Geometry: final body of the model. Coordinates: model frame, mm. Face numbers are marked on the shaded views. A direction names the side the tool comes from. Coordinates: 2 decimals unless noted, no trailing zeros. Write each loop counter-clockwise with the first axis right and the second up, starting at its lowest first coordinate (ties: lowest second). Pieces come first, ordered by that corner, then holes. Notation, with made-up numbers: (-22.75, 60) - (30.25, 60) arc R19 cw to (30.25, 69) - close; hole circle Ø2 at (82, -25). An arc over 180 degrees is marked (long way). Answer as a JSON object with one key per item and string values. Group by question number.
Item 1: First-contact query: pin 1 Ø1.5 at (y, z) = (6.5, 1) entering from +X; pin 2 Ø10 at (x, y) = (0, 0) entering from -Z; pin 3 Ø9.5 at (x, y) = (0, 18.97) entering from -Z; pin 4 Ø3.5 at (y, z) = (26, 3) entering from +X. Flat tips, straight axial feed; report the tip coordinate or a pass-through.
Item 2: Set-up query: the marked faces 5, 6 and 7. Return all of +Z, -Z, +X, -X, +Y, -Y with unobstructed straight access to the full face (end or side cutting, diameter ignored); none if empty.
Item 3: Mould query, pull axis X, two halves, no side actions, for the marked faces 1, 2, 3 and 4. Classes: pulls with the +X half, pulls with the -X half, needs draft (parallel to the pull), parting line crosses it, or undercut.
Item 4: Section A-A on y = 34. Return loops of the section in (x, z).
Item 5: Section B-B on z = 1. State how many separate pieces and enclosed holes the cut face has, and give its area (3 significant figures).
Item 6: Line query: line 1 along Y through (x, z) = (0, 5); line 2 along X through (y, z) = (-4, 6); line 3 along X through (y, z) = (-1, 0.5). Output: solid intervals per line, ascending. Write a range as from..to.
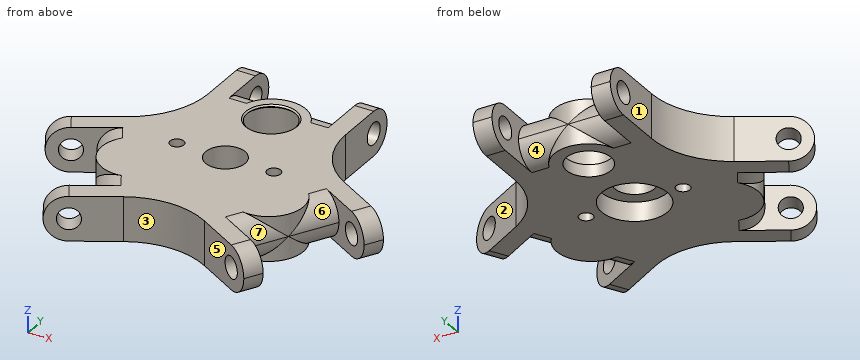
```python
from build123d import *

# Parameters (mm, degrees)
SKETCH1_R           = 8.15
BOSS_EXTRUDE1_DEPTH = 11
FILLET1_R           = 5.5
SKETCH5_R           = 8.534526782
BOSS_EXTRUDE2_DEPTH = 11
SKETCH6_R           = 8.534526782
BOSS_EXTRUDE3_DEPTH = 11
SKETCH7_R           = 8.534526782
BOSS_EXTRUDE4_DEPTH = 11
SKETCH8_R           = 1.7
CUT_EXTRUDE4_DEPTH  = 58.906789501
BOSS_EXTRUDE5_START = -6.25
SKETCH12_R          = 8.15
BOSS_EXTRUDE5_DEPTH = 6.25
SKETCH14_R          = 4.8895
CUT_EXTRUDE7_DEPTH  = 58.906789501
SKETCH15_R          = 6.7
CUT_EXTRUDE8_DEPTH  = 8
SKETCH16_R          = 5.5
CUT_EXTRUDE9_DEPTH  = 58.412509697
SKETCH18_R          = 6.7
SKETCH18_R_2        = 5.95
BOSS_EXTRUDE6_DEPTH = 0.75
CHAMFER1_SIZE       = 0.375
CHAMFER2_SIZE       = 0.375
FILLET2_R           = 5.5
SKETCH19_R          = 2.675
CUT_EXTRUDE10_DEPTH = 72.149372656
SKETCH20_R          = 2.675
CUT_EXTRUDE11_DEPTH = 71.861300583
SKETCH21_R          = 2.675
CUT_EXTRUDE12_DEPTH = 75.055602664


with BuildPart() as part:
    # Sketch1 → Boss-Extrude1 (new body)
    with BuildSketch(Plane.XY):
        with BuildLine():
            Line((-16.980762114, 38.5), (-12.280762114, 38.5))
            Line((-12.280762114, 38.5), (-12.280762114, 27.5))
            Line((-12.280762114, 27.5), (12.280762114, 27.5))
            Line((12.280762114, 27.5), (12.280762114, 38.5))
            Line((12.280762114, 38.5), (16.980762114, 38.5))
            Line((16.980762114, 38.5), (16.980762114, 21.350852961))
            ThreePointArc((16.980762114, 21.350852961), (19.660254038, 11.350852961), (26.980762114, 4.030344885))
            Line((26.980762114, 4.030344885), (41.832359102, -4.544228634))
            Line((41.832359102, -4.544228634), (39.482359102, -8.614548032))
            Line((39.482359102, -8.614548032), (29.956079661, -3.114548032))
            Line((29.956079661, -3.114548032), (17.675317547, -24.385451968))
            Line((17.675317547, -24.385451968), (27.201596989, -29.885451968))
            Line((27.201596989, -29.885451968), (24.851596989, -33.955771366))
            Line((24.851596989, -33.955771366), (10, -25.381197846))
            ThreePointArc((10, -25.381197846), (0, -22.701705922), (-10, -25.381197846))
            Line((-10, -25.381197846), (-24.851596989, -33.955771366))
            Line((-24.851596989, -33.955771366), (-27.201596989, -29.885451968))
            Line((-27.201596989, -29.885451968), (-17.675317547, -24.385451968))
            Line((-17.675317547, -24.385451968), (-29.956079661, -3.114548032))
            Line((-29.956079661, -3.114548032), (-39.482359102, -8.614548032))
            Line((-39.482359102, -8.614548032), (-41.832359102, -4.544228634))
            Line((-41.832359102, -4.544228634), (-26.980762114, 4.030344885))
            ThreePointArc((-26.980762114, 4.030344885), (-19.660254038, 11.350852961), (-16.980762114, 21.350852961))
            Line((-16.980762114, 21.350852961), (-16.980762114, 38.5))
        make_face()
        Circle(SKETCH1_R, mode=Mode.SUBTRACT)
    extrude(amount=BOSS_EXTRUDE1_DEPTH)

    # Fillet1
    fillet1_edges = [part.edges().sort_by_distance(p)[0] for p in [
        (-23.815698604, -13.75, 0),
        (23.815698604, -13.75, 0),
        (23.815698604, -13.75, 11),
        (-23.815698604, -13.75, 11),
        (0, 27.5, 0),
        (0, 27.5, 11),
    ]]
    fillet(fillet1_edges, radius=FILLET1_R - 0.0001)  # a hair under: the kernel refuses the full size

    # Sketch5 → Boss-Extrude2 (add)
    with BuildSketch(Plane(origin=(0, 0, 0), x_dir=(-1, 0, 0), z_dir=(0, 0, -1))):
        with Locations((0, 18.965473218)):
            Circle(SKETCH5_R)
    extrude(amount=-BOSS_EXTRUDE2_DEPTH)

    # Sketch6 → Boss-Extrude3 (add)
    with BuildSketch(Plane(origin=(0, 0, 0), x_dir=(-1, 0, 0), z_dir=(0, 0, -1))):
        with Locations((-16.424581602, -9.482736609)):
            Circle(SKETCH6_R)
    extrude(amount=-BOSS_EXTRUDE3_DEPTH)

    # Sketch7 → Boss-Extrude4 (add)
    with BuildSketch(Plane.XY.offset(11)):
        with Locations((-16.424581602, -9.482736609)):
            Circle(SKETCH7_R)
    extrude(amount=-BOSS_EXTRUDE4_DEPTH)

    # Sketch8 → Cut-Extrude4 (cut, through all)
    with BuildSketch(Plane.XY.offset(11)):
        with Locations((-12, 0)):
            Circle(SKETCH8_R)
        with Locations((12, 0)):
            Circle(SKETCH8_R)
    extrude(amount=-CUT_EXTRUDE4_DEPTH, mode=Mode.SUBTRACT)

    # Sketch12 → Boss-Extrude5 (add)
    with BuildSketch(Plane.XY.offset(11).offset(BOSS_EXTRUDE5_START)):
        Circle(SKETCH12_R)
    extrude(amount=BOSS_EXTRUDE5_DEPTH)

    # Sketch14 → Cut-Extrude7 (cut, through all)
    with BuildSketch(Plane.XY.offset(11)):
        Circle(SKETCH14_R)
    extrude(amount=-CUT_EXTRUDE7_DEPTH, mode=Mode.SUBTRACT)

    # Sketch15 → Cut-Extrude8 (cut)
    with BuildSketch(Plane.XY.offset(11)):
        with Locations((0, 18.965473218)):
            Circle(SKETCH15_R)
    extrude(amount=-CUT_EXTRUDE8_DEPTH, mode=Mode.SUBTRACT)

    # Sketch16 → Cut-Extrude9 (cut, through all)
    with BuildSketch(Plane.XY.offset(3)):
        with Locations((0, 18.965473218)):
            Circle(SKETCH16_R)
    extrude(amount=-CUT_EXTRUDE9_DEPTH, mode=Mode.SUBTRACT)

    # Sketch18 → Boss-Extrude6 (add)
    with BuildSketch(Plane.XY.offset(11)):
        with Locations((0, 18.965473218)):
            Circle(SKETCH18_R)
        with Locations((0, 18.965473218)):
            Circle(SKETCH18_R_2, mode=Mode.SUBTRACT)
    extrude(amount=-BOSS_EXTRUDE6_DEPTH)

    # Chamfer1
    chamfer1_edges = [part.edges().sort_by_distance(p)[0] for p in [
        (-5.95, 18.965473218, 11),
    ]]
    chamfer(chamfer1_edges, length=CHAMFER1_SIZE)

    # Chamfer2
    chamfer2_edges = [part.edges().sort_by_distance(p)[0] for p in [
        (-5.95, 18.965473218, 10.25),
    ]]
    chamfer(chamfer2_edges, length=CHAMFER2_SIZE - 0.0001)  # a hair under: the kernel refuses the full size

    # Fillet2
    fillet2_edges = [part.edges().sort_by_distance(p)[0] for p in [
        (26.026596989, -31.920611667, 0),
        (40.657359102, -6.579388333, 0),
        (26.026596989, -31.920611667, 11),
        (40.657359102, -6.579388333, 11),
        (14.630762114, 38.5, 0),
        (14.630762114, 38.5, 11),
        (-40.657359102, -6.579388333, 0),
        (-40.657359102, -6.579388333, 11),
        (-26.026596989, -31.920611667, 0),
        (-26.026596989, -31.920611667, 11),
        (-14.630762114, 38.5, 0),
        (-14.630762114, 38.5, 11),
    ]]
    fillet(fillet2_edges, radius=FILLET2_R - 0.0001)  # a hair under: the kernel refuses the full size

    # Sketch19 → Cut-Extrude10 (cut, through all)
    with BuildSketch(Plane.ZY.offset(16.980762114)):
        with Locations(Location((5.5, 33, 0), (0, 0, 270))):
            Circle(SKETCH19_R)
    extrude(amount=-CUT_EXTRUDE10_DEPTH, mode=Mode.SUBTRACT)

    # Sketch20 → Cut-Extrude11 (cut, through all)
    with BuildSketch(Plane(origin=(-8.490381057, 14.705771366, 0), x_dir=(0.8660254037844307, 0.5000000000000139, 0), z_dir=(-0.5000000000000139, 0.8660254037844307, 0))):
        with Locations((-33, -5.5)):
            Circle(SKETCH20_R)
    extrude(amount=-CUT_EXTRUDE11_DEPTH, mode=Mode.SUBTRACT)

    # Sketch21 → Cut-Extrude12 (cut, through all)
    with BuildSketch(Plane(origin=(-8.490381057, -14.705771366, 0), x_dir=(0.8660254037844329, -0.50000000000001, 0), z_dir=(-0.5000000000000099, -0.8660254037844328, 0))):
        with Locations(Location((33, 5.5, 0), (0, 0, 180))):
            Circle(SKETCH21_R)
    extrude(amount=-CUT_EXTRUDE12_DEPTH, mode=Mode.SUBTRACT)


solid = part.part
```
Checks:
{
 "1": {"pin 1": "x = 24.47", "pin 2": "z = 4.75", "pin 3": "through", "pin 4": "x = 16.98"},
 "2": {"face 5": "+Z, -Z, -Y", "face 6": "+Z", "face 7": "+Z, +X"},
 "3": {"face 1": "pulls with the -X half", "face 2": "pulls with the +X half", "face 3": "undercut", "face 4": "undercut"},
 "4": {"outline": "(-16.98, 0.09) - (-12.28, 0.09) - (-12.28, 3.02) - (-16.98, 3.02) - close; (-16.98, 7.98) - (-12.28, 7.98) - (-12.28, 10.91) - (-16.98, 10.91) - close; (12.28, 0.09) - (16.98, 0.09) - (16.98, 3.02) - (12.28, 3.02) - close; (12.28, 7.98) - (16.98, 7.98) - (16.98, 10.91) - (12.28, 10.91) - close"},
 "5": {"separate pieces": "1", "enclosed holes": "4", "area": "2,170 mm^2"},
 "6": {"line 1": "-22.7..-4.89, 4.89..12.27, 25.67..27.5", "line 2": "-40.89..-38.83, -32.76..-31.49, -29.42..-2.81, 2.81..29.42, 31.49..32.76, 38.83..40.89", "line 3": "-35.69..-13.37, -10.63..-8.09, 8.09..10.63, 13.37..35.69"}
}
